For this review, take the finished solid that the model builds, in its own axes (mm). A direction names the side the tool comes from. Coordinates: 2 decimals unless noted, no trailing zeros. Order: outer loops, then holes, each group sorted by start corner. A loop starts at its lowest first (then second) coordinate and runs counter-clockwise, first axis right, second up. Notation, with made-up numbers: M 58.25,43.25 L 106.25,43.25 A12 cw 106.25,63.25 Z; hole C 0,-16 d7. An arc over 180 degrees is marked long. Use one line per item in the form item = value. Start each with the question number.
```python
from build123d import *

# Parameters (mm, degrees)
F0_W     = 94
F0_H     = 74
F0_W_2   = 92
F0_H_2   = 72
F1_DEPTH = 4
F0_W_3   = 86
F0_H_3   = 66
F2_DEPTH = 1


with BuildPart() as f1:
    # F0 (on Top) → F1 (new body)
    with BuildSketch(Plane.XY):
        Rectangle(F0_W, F0_H)
        Rectangle(F0_W_2, F0_H_2, mode=Mode.SUBTRACT)
    extrude(amount=F1_DEPTH)

    # F0 (on Top) → F2 (join)
    with BuildSketch(Plane.XY):
        Rectangle(F0_W_2, F0_H_2)
        Rectangle(F0_W_3, F0_H_3, mode=Mode.SUBTRACT)
    extrude(amount=F2_DEPTH)


solid = f1.part
```
1. The part is to be moulded in two halves that separate along Y. For faces 3 (the flat face through (-1, 37, 2)), 4 (the flat face through (47, -1, 2)), 5 (the flat face through (46, -1, 2)), say which applies: pulls with the +Y half, pulls with the -Y half, needs draft (parallel to the pull), parting line crosses it, or undercut.
2. To check wall thickness, follow line 1 (Y direction, x = -2, z = 2.45); line 2 (X direction, y = -17.5, z = 0.4); line 3 (X direction, y = -21, z = 2.8). State the ranges of each line that lie inside material, in increasing order.
3. Consider section B-B, the plane x = -0.5. Write out the cut boundary in (y, z), plus the area to 3 significant figures.
4. Consider section A-A, the plane y = -10. Write out the cut boundary in (x, z).
5. Consider section C-C, the plane z = 3. Write out the cut boundary in (x, y), plus the area to 3 significant figures.
6. Tool access review of faces 1 (the flat face through (-1, -36, 2)), 2 (the flat face through (-1, -37, 2)): name each direction out of +Z, -Z, +X, -X, +Y, -Y from which nothing blocks a thin tool from reaching the whole face with its end or side.
Answers follow:
q1.face_3 = pulls with the +Y half
q1.face_4 = needs draft
q1.face_5 = undercut
q2.line_1 = -37 to -36, 36 to 37
q2.line_2 = -47 to -43, 43 to 47
q2.line_3 = -47 to -46, 46 to 47
q3.outline = M -37,0 L -33,0 L -33,1 L -36,1 L -36,4 L -37,4 Z; M 33,0 L 37,0 L 37,4 L 36,4 L 36,1 L 33,1 Z
q3.area = 14.0 mm²
q4.outline = M -47,0 L -43,0 L -43,1 L -46,1 L -46,4 L -47,4 Z; M 43,0 L 47,0 L 47,4 L 46,4 L 46,1 L 43,1 Z
q5.outline = M -47,-37 L 47,-37 L 47,37 L -47,37 Z; hole M -46,-36 L 46,-36 L 46,36 L -46,36 Z
q5.area = 332 mm²
q6.face_1 = +Z
q6.face_2 = +Z, -Z, +X, -X, -Y
